Check sheet for the drawn part. Datum: minimum x, y, z corner. Units: mm. Coordinates: 2 decimals unless noted, no trailing zeros. Order: outer loops, then holes, each group sorted by start corner. A loop starts at its lowest first (then second) coordinate and runs counter-clockwise, first axis right, second up.
Q1. Thickness scan on line 1 (X direction, y = 7.5, z = 19) (1 decimal); line 2 (X direction, y = 5.25, z = 16); line 3 (Z direction, x = 20, y = 1.25) (1 decimal). Record the ranges inside material, lowest first.
Q2. Cross-section at D-D, the plane x = 27. Record the boundary of the cut face in (y, z), and give its area (3 significant figures).
Q3. Cross-section at C-C, the plane x = 9.5. Record the boundary of the cut face in (y, z) (1 decimal).
Q4. Depth check by flat-ended pin: P1, Ø5, axis at x = 10.5, y = 2, coming from the -Z side (1 decimal). Enter the tip coordinate at first touch or a pass-through.
Q5. Cross-section at A-A, the plane z = 19. Record the boundary of the cut face in (x, y) (1 decimal).
Q6. Cross-section at B-B, the plane y = 10.5. Record the boundary of the cut face in (x, z) (1 decimal).
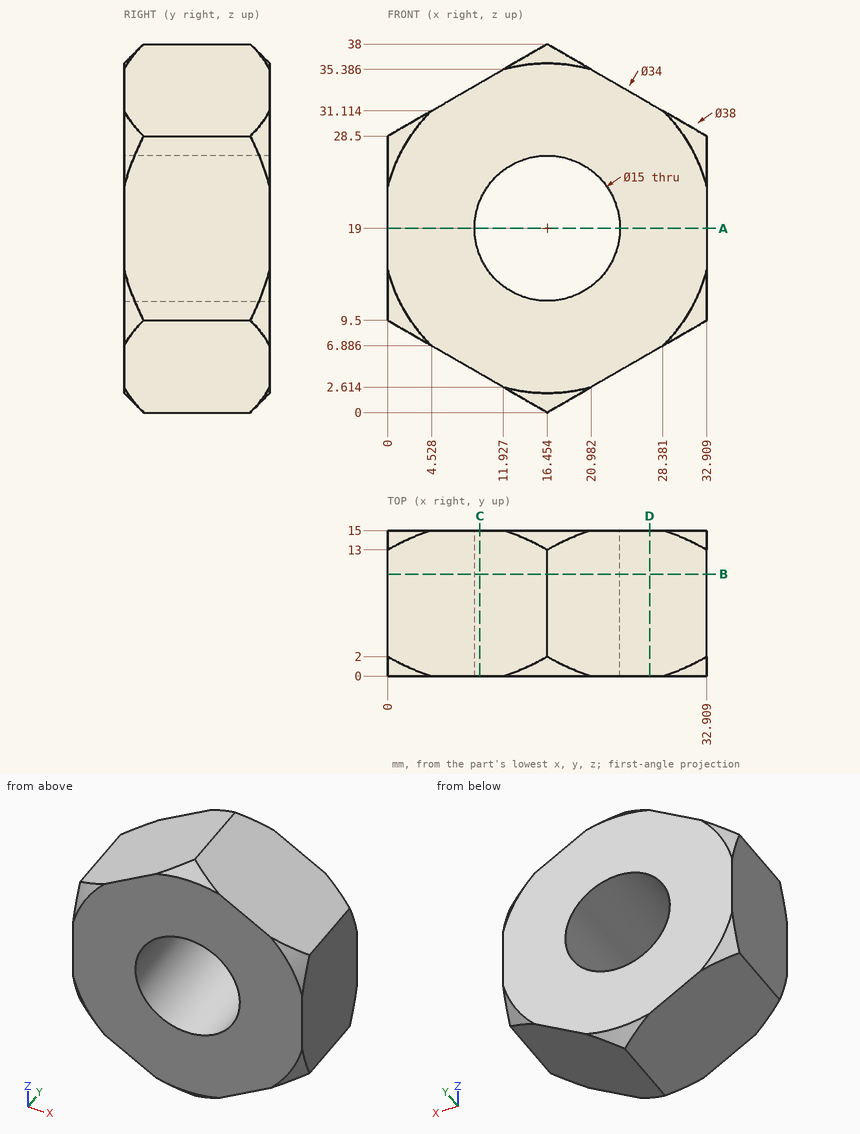
Check values:
1. line 1: x = 0 to 9, 24 to 32.9
1. line 2: x = 0 to 9.58, 23.33 to 32.91
1. line 3: z = 2 to 12.4, 25.6 to 36
2. outline: (0, 6.09) - (15, 6.09) - (15, 31.91) - (0, 31.91) - close
2. area: 387 mm2
3. outline: (0, 4) - (15, 4) - (15, 16.2) - (0, 16.2) - close; (0, 21.8) - (15, 21.8) - (15, 34) - (0, 34) - close
4. P1: stops at z = 2
5. outline: (0, 0) - (9, 0) - (9, 15) - (0, 15) - close; (24, 0) - (32.9, 0) - (32.9, 15) - (24, 15) - close
6. outline: (0, 9.5) - (16.5, 0) - (32.9, 9.5) - (32.9, 28.5) - (16.5, 38) - (0, 28.5) - close; hole circle Ø15 at (16.5, 19)
